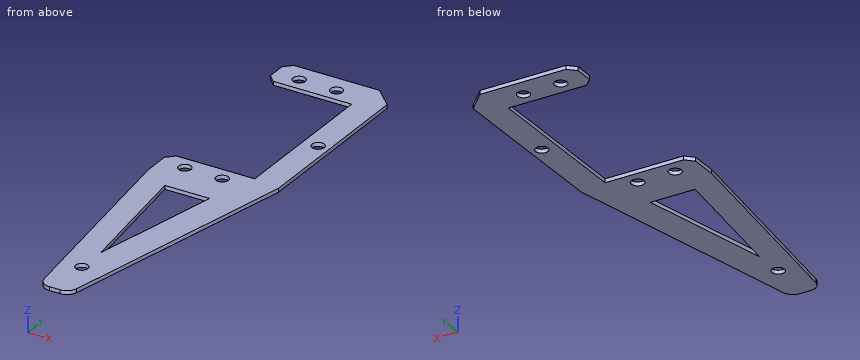
from build123d import *

# Parameters (mm, degrees)
SM_BASE_FLANGE_1_DEPTH  = 1
HOLE_WIZARD_3_3_3_3_1_D = 3.3
CHAMFER_2_SIZE          = 5
FILLET_1_R              = 3
CHAMFER_3_SIZE          = 2


# Sheet-metal steps are written as plain solids
with BuildPart() as part:
    # Sketch 1 → 基体-法兰1 (new body)
    with BuildSketch(Plane.XY):
        Polygon((-23, 0), (0, 0), (0, 42.2), (-23, 42.2), (-23, 51.2), (7, 51.2), (7, -1.053326424), (-7.4, -68.8), (-15.4, -68.8), (-23, -9), align=None)
        Polygon((-15.817797263, -13.469186385), (-3.817797263, -13.469186385), (-11.327593526, -48.8), align=None, mode=Mode.SUBTRACT)
    extrude(amount=-SM_BASE_FLANGE_1_DEPTH)

    # Ø3.3 (3.3) 直径孔1 (through all)
    with Locations(Plane.XY):
        with Locations((-6.4, 46), (-16.4, 46), (-16.4, -3.8), (-6.4, -3.8), (4, 21.1), (-11.4, -56.8)):
            Hole(HOLE_WIZARD_3_3_3_3_1_D / 2)

    # 倒角2
    chamfer_2_edges = [part.edges().sort_by_distance(p)[0] for p in [
        (7, 51.2, -0.5),
    ]]
    chamfer(chamfer_2_edges, length=CHAMFER_2_SIZE)

    # 圆角1
    fillet_1_edges = [part.edges().sort_by_distance(p)[0] for p in [
        (-7.4, -68.8, -0.5),
        (-15.4, -68.8, -0.5),
    ]]
    fillet(fillet_1_edges, radius=FILLET_1_R)

    # 倒角3
    chamfer_3_edges = [part.edges().sort_by_distance(p)[0] for p in [
        (-23, 0, -0.5),
        (-23, 42.2, -0.5),
        (-23, 51.2, -0.5),
    ]]
    chamfer(chamfer_3_edges, length=CHAMFER_3_SIZE)


solid = part.part
Geometry check sheet. Reference: the model listing, model coordinates, mm. Round coordinates to 2 decimals unless told otherwise and drop trailing zeros. Order: outer loops, then holes, each group sorted by start corner. A loop starts at its lowest first (then second) coordinate and runs counter-clockwise, first axis right, second up. Notation, with made-up numbers: (-36, 20) - (-32, 20) arc R22 ccw to (-32, 30) - close; hole circle Ø1 at (89.5, 55.5). An arc over 180 degrees is marked (long way). One line per question, with ' | ' between items. Start each with the question number.
(1) Depth check by flat-ended pin: pin 1 Ø3 at (x, y) = (4, 21.1) entering from -Z (3 decimals); pin 2 Ø4 at (x, y) = (-6.4, 46) entering from -Z. Enter the tip coordinate at first touch or a pass-through.
(2) Thickness scan on L1, parallel to X at y = 32, z = -0.1; L2, parallel to X at y = -37, z = -0.65; L3, parallel to X at y = -54.5, z = -0.8. Record the ranges inside material, lowest first. Write a range as [from, to].
(3) Sectioned sample at D-D on y = -3.8. Record the cut outline in (x, z), and give its area (3 significant figures).
(4) Sectioned sample at A-A on y = 21.1. Record the cut outline in (x, z), and give its area (3 significant figures).
(5) Sectioned sample at C-C on x = 4. Record the cut outline in (y, z).
(6) Sectioned sample at B-B on z = -0.35. Record the cut outline in (x, y), and give its area (3 significant figures).
Conclusion:
1) pin 1: passes through | pin 2: stops at z = -1
2) L1: x = [0, 7] | L2: x = [-19.44, -12.83], [-8.82, -0.64] | L3: x = [-17.22, -4.36]
3) outline: (-23, -1) - (-18.05, -1) - (-18.05, 0) - (-23, 0) - close; (-14.75, -1) - (-8.05, -1) - (-8.05, 0) - (-14.75, 0) - close; (-4.75, -1) - (6.42, -1) - (6.42, 0) - (-4.75, 0) - close | area: 22.8 mm2
4) outline: (0, -1) - (2.35, -1) - (2.35, 0) - (0, 0) - close; (5.65, -1) - (7, -1) - (7, 0) - (5.65, 0) - close | area: 3.70 mm2
5) outline: (-15.17, -1) - (19.45, -1) - (19.45, 0) - (-15.17, 0) - close; (22.75, -1) - (49.2, -1) - (49.2, 0) - (22.75, 0) - close
6) outline: (-23, -9) - (-15.73, -66.18) arc R3 ccw to (-12.76, -68.8) - (-9.83, -68.8) arc R3 ccw to (-6.89, -66.42) - (7, -1.05) - (7, 46.2) - (2, 51.2) - (-21, 51.2) - (-23, 49.2) - (-23, 44.2) - (-21, 42.2) - (0, 42.2) - (0, 0) - (-21, 0) - (-23, -2) - close; hole circle Ø3.3 at (-16.4, -3.8); hole circle Ø3.3 at (-16.4, 46); hole (-15.82, -13.47) - (-11.33, -48.8) - (-3.82, -13.47) - close; hole circle Ø3.3 at (-11.4, -56.8); hole circle Ø3.3 at (-6.4, -3.8); hole circle Ø3.3 at (-6.4, 46); hole circle Ø3.3 at (4, 21.1) | area: 1,630 mm2
